from build123d import *

# Parameters (mm, degrees)
SKETCH1_W           = 150
SKETCH1_H           = 50
BOSS_EXTRUDE1_DEPTH = 10
SKETCH2_R           = 10
BOSS_EXTRUDE2_DEPTH = 50
SKETCH3_R           = 5
CUT_EXTRUDE1_DEPTH  = 51


with BuildPart() as part:
    # Sketch1 → Boss-Extrude1 (new body)
    with BuildSketch(Plane(origin=(0, 0, 0), x_dir=(1, 0, 0), z_dir=(0, 1, 0))):
        with Locations((-75, 25)):
            Rectangle(SKETCH1_W, SKETCH1_H)
    extrude(amount=BOSS_EXTRUDE1_DEPTH)

    # Sketch2 → Boss-Extrude2 (add, through all)
    with BuildSketch(Plane.XY):
        with Locations((0, 5)):
            Circle(SKETCH2_R)
    extrude(amount=-BOSS_EXTRUDE2_DEPTH)

    # Sketch3 → Cut-Extrude1 (cut, through all)
    with BuildSketch(Plane.XY):
        with Locations((0, 5)):
            Circle(SKETCH3_R)
    extrude(amount=-CUT_EXTRUDE1_DEPTH, mode=Mode.SUBTRACT)


solid = part.part
The listing builds one solid part. Answer for the finished solid, in the listing's coordinates (mm). A direction names the side the tool comes from. Round coordinates to 2 decimals unless told otherwise and drop trailing zeros. Write each loop counter-clockwise with the first axis right and the second up, starting at its lowest first coordinate (ties: lowest second). Pieces come first, ordered by that corner, then holes. Notation, with made-up numbers: (8.5, -7) - (44.5, -7) arc R16 ccw to (44.5, 9) - close; hole circle Ø5 at (81, 2.25). An arc over 180 degrees is marked (long way). Use a Markdown table: item, result. Add a question column.
1. Flat-ended cylindrical pins translate along their axes: P1, Ø2, axis at x = -128.5, z = -45, coming from the +Y side; P2, Ø3, axis at y = 2.5, z = -8.5, coming from the +X side; P3, Ø15, axis at x = -84, z = -34.5, coming from the -Y side. Find the tip coordinate at first contact, or state that the pin passes through.
2. The part is cut by section A-A (x = 0). Write down the section's boundary in (y, z).
3. For a pull along Y with two mould halves and no side action, classify faces 3 (the face through (-80, 10, -25)), 4 (the face through (-71, 5, 0)), 5 (the face through (-1.08, 0.12, -24.65)) as +Y half, -Y half, draft (parallel to the pull), parting line (faces both ways), or undercut.
4. Consider line 1 (Y direction, x = -13, z = -21); line 2 (Y direction, x = 3, z = -5); line 3 (X direction, y = 9, z = -9.5). Determine where each line is inside the solid, lowest interval first.
5. The part is cut by section B-B (y = 5). Write down the section's boundary in (x, z), and give its area (3 significant figures).
6. The part is cut by section D-D (x = -130). Write down the section's boundary in (y, z), and give its area (3 significant figures).
7. The part is cut by section C-C (z = -29). Write down the section's boundary in (x, y), and give its area (3 significant figures).
8. A tool of negligible diameter and unlimited length cuts with its end or side. For faces 1 (the face through (-150, 5, -25)), 2 (the face through (-80, 0, -25)), from which of +Z, -Z, +X, -X, +Y, -Y can it reach the whole face along a straight path? Write none if from no direction.
Reported:
| question | item | result |
|---|---|---|
| 1 | P1 | y = 10 |
| 1 | P2 | x = 9.95 |
| 1 | P3 | y = 0 |
| 2 | outline | (-5, -50) - (0, -50) - (0, 0) - (-5, 0) - close; (10, -50) - (15, -50) - (15, 0) - (10, 0) - close |
| 3 | face 3 | +Y half |
| 3 | face 4 | draft |
| 3 | face 5 | undercut |
| 4 | line 1 | 0 to 10 |
| 4 | line 2 | -4.54 to 1, 9 to 14.54 |
| 4 | line 3 | -150 to -3, 3 to 9.17 |
| 5 | outline | (-150, -50) - (-5, -50) - (-5, 0) - (-150, 0) - close; (5, -50) - (10, -50) - (10, 0) - (5, 0) - close |
| 5 | area | 7,500 mm^2 |
| 6 | outline | (0, -50) - (10, -50) - (10, 0) - (0, 0) - close |
| 6 | area | 500 mm^2 |
| 7 | outline | (-150, 0) - (-8.66, 0) arc R10 ccw (long way) to (-8.66, 10) - (-150, 10) - close; hole circle Ø10 at (0, 5) |
| 7 | area | 1,640 mm^2 |
| 8 | face 1 | +Z, -Z, -X, +Y, -Y |
| 8 | face 2 | +Z, -Z, -X, -Y |
